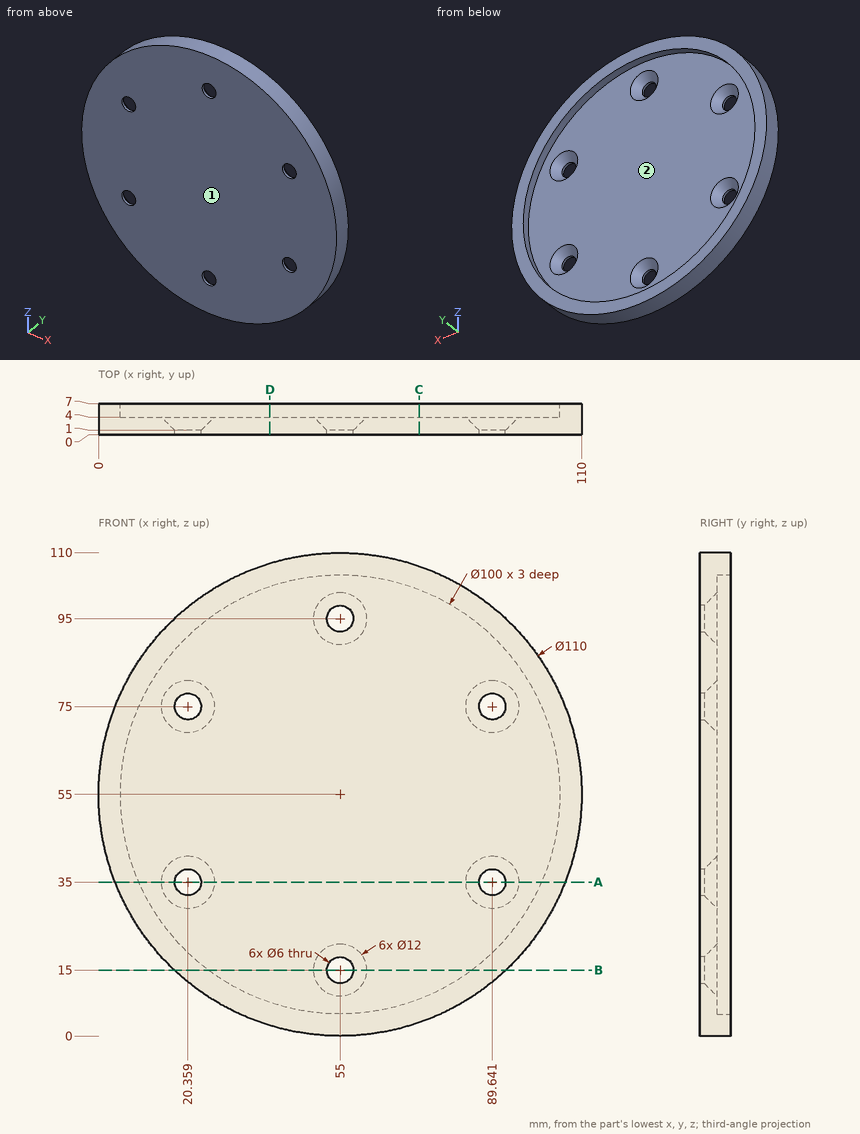
Design review of the part shown in the three views and the two pictorial views. Dimensions are in mm from the part's minimum x, y and z. Round coordinates to 2 decimals unless told otherwise and drop trailing zeros. Loops run counter-clockwise (first coordinate to the right, second up) from the corner with the lowest first, then second, coordinate; pieces in that order, holes last. Notation, with made-up numbers: (63.25, 23.25) - (82.25, 23.25) arc R11 cw to (82.25, 41.25) - close; hole circle Ø10 at (-8, 35). An arc over 180 degrees is marked (long way). Answer as CSV lines item,"result".
(1) Consider section A-A on z = 35. Give the boundary of the cut face in (x, y), then the cut area to 3 significant figures.
Checked values:
outline,"(3.77, 0) - (17.36, 0) - (17.36, 1) - (14.36, 4) - (9.17, 4) - (9.17, 7) - (3.77, 7) - close; (23.36, 0) - (86.64, 0) - (86.64, 1) - (83.64, 4) - (26.36, 4) - (23.36, 1) - close; (92.64, 0) - (106.23, 0) - (106.23, 7) - (100.83, 7) - (100.83, 4) - (95.64, 4) - (92.64, 1) - close"
area,"376 mm2"
(2) Insertion check: P1, Ø3, axis at x = 44, y = 4, coming from the -Z side; P2, Ø2, axis at y = 6, z = 12.5, coming from the -X side; P3, Ø7, axis at x = 89.64, z = 35, coming from the +Y side. Each pin has a flat end and moves straight along its axis. Give the tip position at first contact, or say it passes through.
Checked values:
P1,"stops at z = 0.83"
P2,"stops at x = 18.91"
P3,"stops at y = 1.5"
(3) Consider section C-C on x = 73. Give the boundary of the cut face in (y, z).
Checked values:
outline,"(0, 3.03) - (7, 3.03) - (7, 8.35) - (4, 8.35) - (4, 101.65) - (7, 101.65) - (7, 106.97) - (0, 106.97) - close"
(4) Consider section D-D on x = 39. Give the boundary of the cut face in (y, z).
Checked values:
outline,"(0, 2.38) - (7, 2.38) - (7, 7.63) - (4, 7.63) - (4, 102.37) - (7, 102.37) - (7, 107.62) - (0, 107.62) - close"
(5) Wall thickness on line 1 (X direction, y = 0.25, z = 35); line 2 (Z direction, x = 20.5, y = 2.25); line 3 (Z direction, x = 88, y = 3.5): over which ranges is each line inside the solid? List them lowest first.
Checked values:
line 1,"x = 3.77 to 17.36, 23.36 to 86.64, 92.64 to 106.23"
line 2,"z = 12.17 to 30.75, 39.25 to 70.75, 79.25 to 97.83"
line 3,"z = 11 to 29.75, 40.25 to 69.75, 80.25 to 99"
(6) Mouldability with a two-part tool opening along Z and no side actions: class the marked faces 1 and 2 as +Z half, -Z half, draft (parallel to the pull), parting line (faces both ways), or undercut.
Checked values:
face 1,"draft"
face 2,"undercut"
(7) Consider section B-B on z = 15. Give the boundary of the cut face in (x, y).
Checked values:
outline,"(17.25, 0) - (52, 0) - (52, 1) - (49, 4) - (25, 4) - (25, 7) - (17.25, 7) - close; (58, 0) - (92.75, 0) - (92.75, 7) - (85, 7) - (85, 4) - (61, 4) - (58, 1) - close"
